from build123d import *

# Parameters (mm, degrees)
F0_R     = 12.7
F1_DEPTH = 25.4
F3_DEPTH = 25.4
F4_R     = 5.08


with BuildPart() as f1:
    # F0 (on Front) → F1 (new body)
    with BuildSketch(Plane.XZ):
        with BuildLine():
            Line((57.099202013, -20.9237289011), (-30.2629248588, 38.2105994406))
            ThreePointArc((-30.2629248588, 38.2105994406), (-56.4070573186, 39.6128704117), (-69.900797987, 17.1762710989))
            Line((-69.900797987, 17.1762710989), (-69.900797987, -33.6237289011))
            Line((-69.900797987, -33.6237289011), (57.099202013, -33.6237289011))
            Line((57.099202013, -33.6237289011), (57.099202013, -20.9237289011))
        make_face()
        with Locations((-44.500797987, 17.1762710989)):
            Circle(F0_R, mode=Mode.SUBTRACT)
    extrude(amount=F1_DEPTH)

    # F2 (on face) → F3 (join)
    with BuildSketch(Plane.XZ.offset(25.4)):
        with BuildLine():
            Line((-19.100797987, -20.9237289011), (-19.100797987, 17.1762710989))
            Line((-19.100797987, 17.1762710989), (-31.800797987, 17.1762710989))
            ThreePointArc((-31.800797987, 17.1762710989), (-44.500797987, 4.4762710989), (-57.200797987, 17.1762710989))
            Line((-57.200797987, 17.1762710989), (-69.900797987, 17.1762710989))
            Line((-69.900797987, 17.1762710989), (-69.900797987, -20.9237289011))
            Line((-69.900797987, -20.9237289011), (-69.900797987, -33.6237289011))
            Line((-69.900797987, -33.6237289011), (57.099202013, -33.6237289011))
            Line((57.099202013, -33.6237289011), (57.099202013, -20.9237289011))
            Line((57.099202013, -20.9237289011), (-19.100797987, -20.9237289011))
        make_face()
        with BuildLine():
            Line((-31.800797987, 17.1762710989), (-19.100797987, 17.1762710989))
            ThreePointArc((-19.100797987, 17.1762710989), (-22.0641986741, 29.0825304305), (-30.2629248588, 38.2105994406))
            ThreePointArc((-30.2629248588, 38.2105994406), (-56.4070573186, 39.6128704117), (-69.900797987, 17.1762710989))
            Line((-69.900797987, 17.1762710989), (-57.200797987, 17.1762710989))
            ThreePointArc((-57.200797987, 17.1762710989), (-44.500797987, 29.8762710989), (-31.800797987, 17.1762710989))
        make_face()
    extrude(amount=F3_DEPTH)

    # F4
    f4_edges = [f1.edges().sort_by_distance(p)[0] for p in [
        (57.099202, -50.8, -27.273729),
    ]]
    fillet(f4_edges, radius=F4_R)


solid = f1.part
Verification items for the finished model (mm, model axes). A direction names the side the tool comes from. Give positions to 0.01 mm unless a question says otherwise; leave off trailing zeros. Loops run counter-clockwise (first coordinate to the right, second up) from the corner with the lowest first, then second, coordinate; pieces in that order, holes last.
1) Sectioned sample at D-D, the plane y = -5.5. Enter the section's corners in (x, z), then the cut area to 3 significant figures.
2) Thickness scan on line 1 along Z through (x, y) = (-44, -28); line 2 along Z through (x, y) = (34, -25.5); line 3 along X through (y, z) = (-32, 14). Record the ranges inside material, lowest first.
3) Depth check by flat-ended pin: pin 1 Ø1.5 at (y, z) = (-27, -3) entering from +X; pin 2 Ø20.5 at (x, y) = (35, -43.5) entering from +Z; pin 3 Ø5 at (x, y) = (-19, -41) entering from +Z. Enter the tip coordinate at first touch or a pass-through.
4) Sectioned sample at B-B, the plane z = 14. Enter the section's corners in (x, y).
5) Draft check along Y on faces 3 (the flat face through (-21, 0, -3)), 4 (the flat face through (-37, -50.8, -3)), 5 (the flat face through (14.03, -12.52, 8.23)). Enter one of: pulls with the +Y half, pulls with the -Y half, needs draft (parallel to the pull), parting line crosses it, or undercut.
6) Sectioned sample at A-A, the plane y = -32. Enter the section's corners in (x, z), then the cut area to 3 significant figures.
7) Set-up check for faces 1 (the flat face through (-19.101, -38, -2)), 2 (the flat face through (-69.901, -25, -8)): record each of +Z, -Z, +X, -X, +Y, -Y from which the full face is reachable in a straight line by a thin tool's end or side.
8) Sectioned sample at C-C, the plane x = -47.5. Enter the section's corners in (y, z), then the cut area to 3 significant figures.
Answers:
1. outline: (-69.9, -33.62) - (57.1, -33.62) - (57.1, -20.92) - (-30.26, 38.21) arc R25.4 ccw to (-69.9, 17.18) - close; hole circle Ø25.4 at (-44.5, 17.18)
1. area: 6,050 mm2
2. line 1: z = -33.62 to 4.49, 29.87 to 42.57
2. line 2: z = -33.62 to -20.92
2. line 3: x = -69.9 to -56.8, -32.2 to -19.1
3. pin 1: stops at x = -19.1
3. pin 2: stops at z = -20.92
3. pin 3: stops at z = 27.95
4. outline: (-69.9, -50.8) - (-56.8, -50.8) - (-56.8, 0) - (-69.9, 0) - close; (-32.2, -50.8) - (-19.1, -50.8) - (-19.1, -25.4) - (5.5, -25.4) - (5.5, 0) - (-32.2, 0) - close
5. face 3: pulls with the +Y half
5. face 4: pulls with the -Y half
5. face 5: needs draft
6. outline: (-69.9, -33.62) - (57.1, -33.62) - (57.1, -20.92) - (-19.1, -20.92) - (-19.1, 17.18) arc R25.4 ccw to (-69.9, 17.18) - close; hole circle Ø25.4 at (-44.5, 17.18)
6. area: 4,060 mm2
7. face 1: +Z, +X, -Y
7. face 2: +Z, -Z, -X, +Y, -Y
8. outline: (-50.8, -33.62) - (0, -33.62) - (0, 4.84) - (-50.8, 4.84) - close; (-50.8, 29.52) - (0, 29.52) - (0, 42.4) - (-50.8, 42.4) - close
8. area: 2,610 mm2
